Verification items for this drawing (mm, ordinates from the low corner). A direction names the side the tool comes from. Give positions to 0.01 mm unless a question says otherwise; leave off trailing zeros. Loops run counter-clockwise (first coordinate to the right, second up) from the corner with the lowest first, then second, coordinate; pieces in that order, holes last. Notation, with made-up numbers: (-16, -25) -> (16, -25) arc R8 cw to (16, -19) -> close; hole circle Ø10 at (88, -32). An arc over 180 degrees is marked (long way). Use one line per item in the form item = value. Start each with the question number.
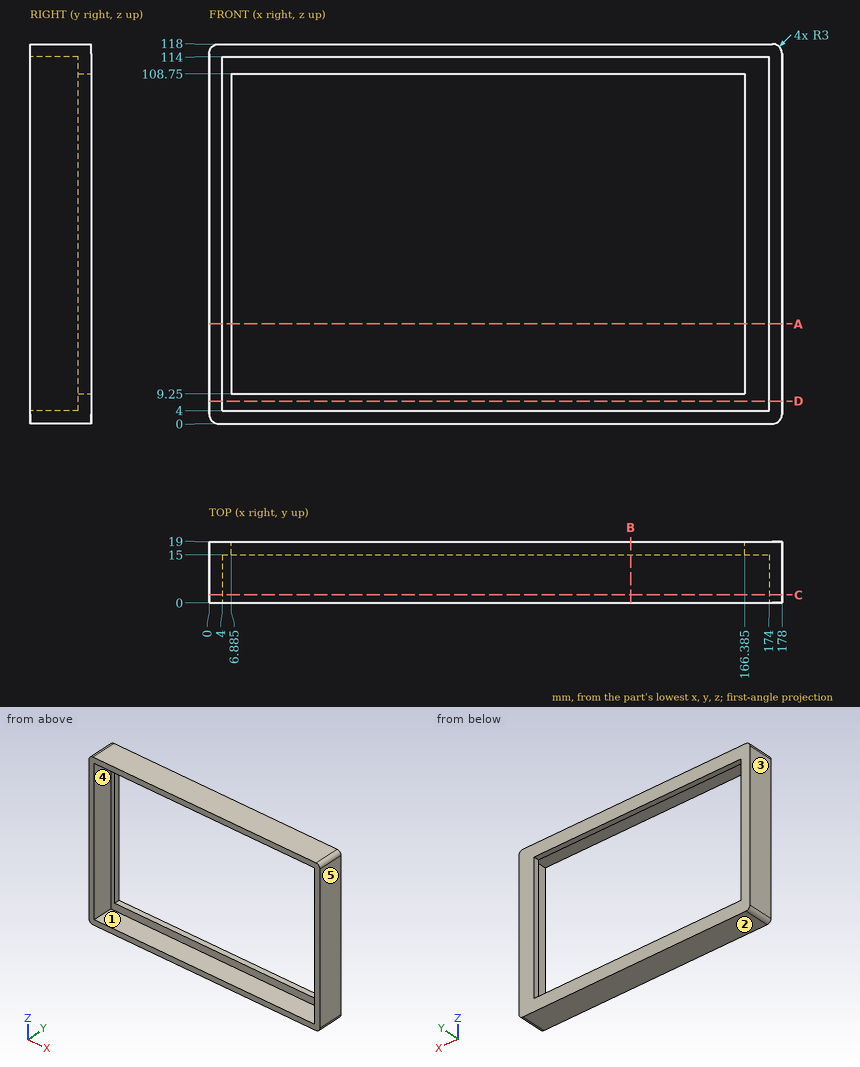
Item 1: Sectioned sample at D-D, the plane z = 7. Enter the section's corners in (x, y), and give its area (3 significant figures).
Item 2: Draft check along X on the marked faces 1, 2 and 3. Enter one of: +X half, -X half, draft (parallel to the pull), parting line (faces both ways), or undercut.
Item 3: Gauge pin test, flat end, axial feed: pin 1 Ø12 at (x, z) = (87, 106) entering from -Y. Record the tip position at first contact, or that the pin passes through.
Item 4: Sectioned sample at A-A, the plane z = 31. Enter the section's corners in (x, y) (1 decimal), and give its area (3 significant figures).
Item 5: Material ranges on line 1 (Z direction, x = 85, y = 8); line 2 (X direction, y = 8, z = 20.5); line 3 (Z direction, x = 83, y = 16.25), recorded low to high.
Item 6: Sectioned sample at B-B, the plane x = 131. Enter the section's corners in (y, z), and give its area (3 significant figures).
Item 7: Tool access check on the marked faces 4 and 5. Record the directions out of +Z, -Z, +X, -X, +Y, -Y that give a thin tool (end or side, any length) a straight path to the whole face; none if there is none.
Item 8: Sectioned sample at C-C, the plane y = 2.5. Enter the section's corners in (x, z).
Outcome:
q1.outline = (0, 0) -> (4, 0) -> (4, 15) -> (174, 15) -> (174, 0) -> (178, 0) -> (178, 19) -> (0, 19) -> close
q1.area = 832 mm^2
q2.face_1 = undercut
q2.face_2 = draft
q2.face_3 = -X half
q3.pin_1 = 15
q4.outline = (0, 0) -> (4, 0) -> (4, 15) -> (6.9, 15) -> (6.9, 19) -> (0, 19) -> close; (166.4, 15) -> (174, 15) -> (174, 0) -> (178, 0) -> (178, 19) -> (166.4, 19) -> close
q4.area = 194 mm^2
q5.line_1 = 0 to 4, 114 to 118
q5.line_2 = 0 to 4, 174 to 178
q5.line_3 = 0 to 9.25, 108.75 to 118
q6.outline = (0, 0) -> (19, 0) -> (19, 9.25) -> (15, 9.25) -> (15, 4) -> (0, 4) -> close; (0, 114) -> (15, 114) -> (15, 108.75) -> (19, 108.75) -> (19, 118) -> (0, 118) -> close
q6.area = 194 mm^2
q7.face_4 = -Y
q7.face_5 = +Z, -Z, +X, +Y, -Y
q8.outline = (0, 3) arc R3 ccw to (3, 0) -> (175, 0) arc R3 ccw to (178, 3) -> (178, 115) arc R3 ccw to (175, 118) -> (3, 118) arc R3 ccw to (0, 115) -> close; hole (4, 4) -> (174, 4) -> (174, 114) -> (4, 114) -> close
